Study the drawing (mm; zero at the part's minimum x, y, z) and answer. A direction names the side the tool comes from. Round coordinates to 2 decimals unless told otherwise and drop trailing zeros. Write each loop counter-clockwise with the first axis right and the second up, starting at its lowest first coordinate (ties: lowest second). Pieces come first, ordered by that corner, then holes.
(1) Find the intervals of material crossed by probe 1 along Y at (x, z) = (17, 35.5); probe 2 along Y at (x, z) = (40, 48); probe 3 along X at (y, z) = (520, 72.5), in increasing order.
(2) A cutting plane is placed at A-A, the plane x = 75. Give the vertices of the cut face in (y, z), and give its area (3 significant figures).
(3) The mould has two halves that part along Y. Classify the marked faces 1, 2 and 3: +Y half, -Y half, draft (parallel to the pull), parting line (faces both ways), or undercut.
(4) A cutting plane is placed at B-B, the plane y = 504.5. Give the vertices of the cut face in (x, z).
(5) For the marked faces 4 and 5, determine the directions among +Z, -Z, +X, -X, +Y, -Y from which every point of the face is accessible in a straight line to the end or side of a thin tool.
(6) A cutting plane is placed at C-C, the plane y = 644. Give the vertices of the cut face in (x, z).
(7) Each of these flat-tipped pins is pushed along its axis until it touches: pin 1 Ø8 at (x, z) = (58.5, 113) entering from -Y; pin 2 Ø10 at (x, y) = (83, 403) entering from +Z; pin 3 Ø2 at (y, z) = (277, 81) entering from -X; pin 4 Ø12 at (x, y) = (42.5, 281.5) entering from +Z. Where does it stop, or does it pass through?
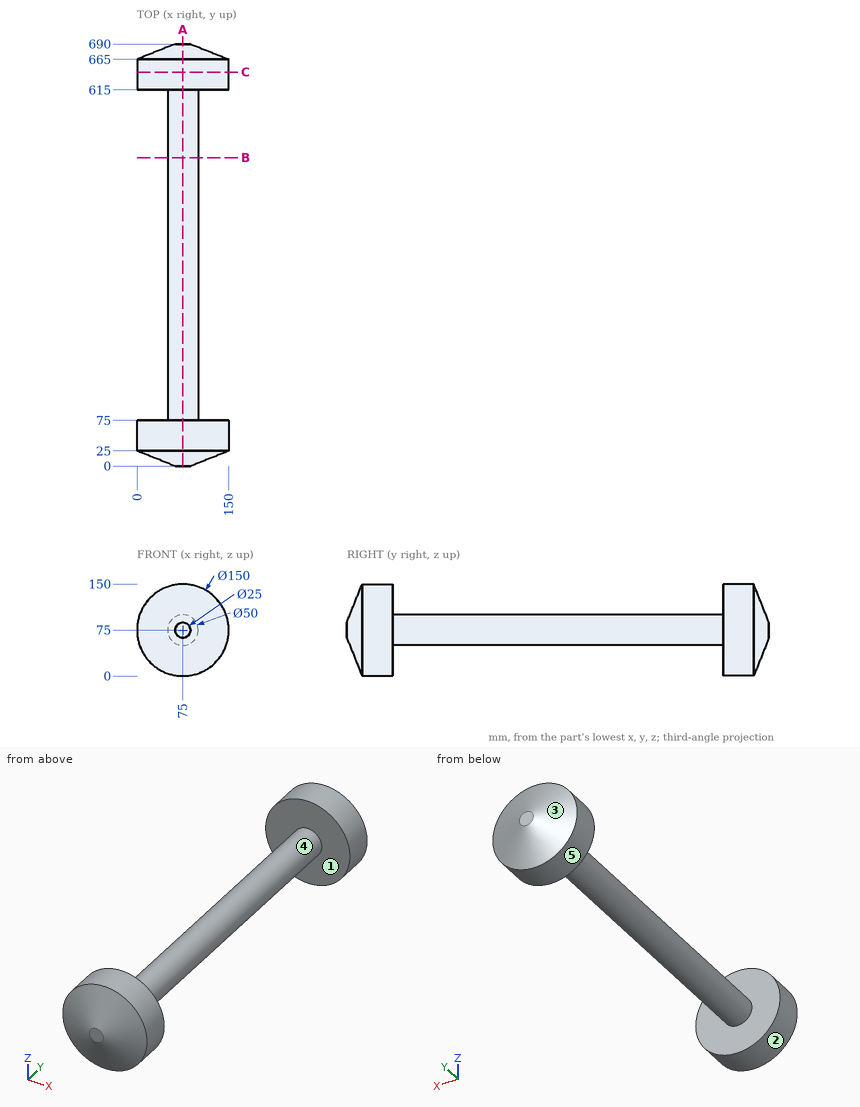
Solutions:
1. probe 1: y = 23.07 to 75, 615 to 666.93
1. probe 2: y = 12.68 to 75, 615 to 677.32
1. probe 3: x = 50.13 to 99.87
2. outline: (0, 62.5) - (25, 0) - (75, 0) - (75, 50) - (615, 50) - (615, 0) - (665, 0) - (690, 62.5) - (690, 87.5) - (665, 150) - (615, 150) - (615, 100) - (75, 100) - (75, 150) - (25, 150) - (0, 87.5) - close
2. area: 46,400 mm2
3. face 1: undercut
3. face 2: draft
3. face 3: +Y half
4. outline: circle Ø50 at (75, 75)
5. face 4: none
5. face 5: +Y, -Y
6. outline: circle Ø150 at (75, 75)
7. pin 1: stops at y = 9.97
7. pin 2: stops at z = 99.82
7. pin 3: stops at x = 50.51
7. pin 4: passes through
